Autodesk Inventor part; units mm, degrees
ref_plane "YZ Plane" through (0, 0, 0) normal (1, 0, 0) x (0, 1, 0)
ref_plane "XZ Plane" through (0, 0, 0) normal (0, 1, 0) x (-1, 0, 0)
ref_plane "XY Plane" through (0, 0, 0) normal (0, 0, 1) x (1, 0, 0)
sketch "Sketch1" plane through (0, 0, 0) normal (0, 0, 1) x (1, 0, 0)
  circle A0 centre (0, 0) radius 37.465
  dimension "d0" = 74.93
extrude "Extrusion1" add sketch "Sketch1" along normal blind 2.54
sketch "Sketch3" plane through (0, 0, 0) normal (0, 0, -1) x (-1, 0, 0)
  circle A0 centre (0, 0) radius 4.191
  circle A1 centre (0, 0) radius 7.9375
  circle A2 centre (0, 0) radius 2.3813
  dimension "d4" = 8.382
  dimension "d5" = 15.875
  dimension "d6" = 4.7625
extrude "Extrusion3" cut sketch "Sketch3" against normal through all contours A0 | A2
extrude "Extrusion4" add sketch "Sketch3" along normal blind 3.81 contours A1
sketch "Sketch4" plane through (0, 0, 2.54) normal (0, 0, 1) x (1, 0, 0)
  line L0 (0, 0) -> (0, 30.48)
  circle A0 centre (0, 30.48) radius 1.5875
  circle A1 centre (-26.3965, 15.24) radius 1.5875
  circle A2 centre (-26.3965, -15.24) radius 1.5875
  circle A3 centre (0, -30.48) radius 1.5875
  circle A4 centre (26.3965, -15.24) radius 1.5875
  circle A5 centre (26.3965, 15.24) radius 1.5875
  dimension "d13" = 30.48
  dimension "d14" = 3.175
  dimension "d17" = 360
extrude "Extrusion5" cut sketch "Sketch4" against normal blind 25.4
properties part number "SpoolEndFrontSide"
Part model, mm, in its own coordinate system. A direction names the side the tool comes from. Round coordinates to 2 decimals unless told otherwise and drop trailing zeros. Order: outer loops, then holes, each group sorted by start corner. A loop starts at its lowest first (then second) coordinate and runs counter-clockwise, first axis right, second up. Notation, with made-up numbers: M 26,21.25 L 40,21.25 A29 cw 40,51.25 Z; hole C -6.75,44 d9. An arc over 180 degrees is marked long. Put each result on its own line as item: value. Start each with the question number.
1. Drop flat-ended pins along their axis: pin 1 (12 mm diameter, centred on x = -8.5, y = -26.5, fed in from -Z); pin 2 (5 mm diameter, centred on x = 0, y = 30.48, fed in from +Z); pin 3 (3 mm diameter, centred on y = -3.5, z = 1, fed in from -X); pin 4 (3 mm diameter, centred on y = -15, z = 0, fed in from -X). Give the stop position or say it passes through.
2. Slice it at A-A on x = 0. List the corners of the cut face in (y, z) (1 decimal), then the cut area to 3 significant figures.
3. Slice it at C-C on y = -30.48. List the corners of the cut face in (x, z).
4. Slice it at D-D on y = 15.24. List the corners of the cut face in (x, z), then the cut area to 3 significant figures.
5. Tool access for faces 4 (the face through (26.1, -16.8, 1.3)), 5 (the face through (1.72, 7.75, -1.88)): list every direction of +Z, -Z, +X, -X, +Y, -Y with a clear straight run to the whole face (end or side of a thin tool).
6. Slice it at B-B on z = 1. List the corners of the cut face in (x, y) (1 decimal).
7. Drill centre lines: probe 1 along Y at (x, z) = (0, 0.5) (1 decimal); probe 2 along Z at (x, y) = (23, -11); probe 3 along Y at (x, z) = (1, 1.25). Where is each one in solid material? Low to high. Write a range as [from, to].
8. Two-plate mould, pull along Y, no slides. Class faces 1 (the face through (8, 1, 2.54)), 2 (the face through (-29.73, 22.8, 1.25)), 3 (the face through (-27.982, 15.31, 1.288)): +Y half, -Y half, draft (parallel to the pull), parting line (faces both ways), or undercut.
Findings:
1. pin 1: z = 0
1. pin 2: z = 2.54
1. pin 3: x = -37.41
1. pin 4: x = -34.95
2. outline: M -37.5,0 L -32.1,0 L -32.1,2.5 L -37.5,2.5 Z; M -28.9,0 L -7.9,0 L -7.9,-3.8 L -4.2,-3.8 L -4.2,2.5 L -28.9,2.5 Z; M 4.2,-3.8 L 7.9,-3.8 L 7.9,0 L 28.9,0 L 28.9,2.5 L 4.2,2.5 Z; M 32.1,0 L 37.5,0 L 37.5,2.5 L 32.1,2.5 Z
2. area: 181 mm2
3. outline: M -21.79,0 L -1.59,0 L -1.59,2.54 L -21.79,2.54 Z; M 1.59,0 L 21.79,0 L 21.79,2.54 L 1.59,2.54 Z
4. outline: M -34.23,0 L -27.98,0 L -27.98,2.54 L -34.23,2.54 Z; M -24.81,0 L 24.81,0 L 24.81,2.54 L -24.81,2.54 Z; M 27.98,0 L 34.23,0 L 34.23,2.54 L 27.98,2.54 Z
4. area: 158 mm2
5. face 4: +Z, -Z
5. face 5: -Z
6. outline: C 0,0 d74.9; hole C -26.4,-15.2 d3.2; hole C -26.4,15.2 d3.2; hole C 0,0 d8.4; hole C 0,-30.5 d3.2; hole C 0,30.5 d3.2; hole C 26.4,-15.2 d3.2; hole C 26.4,15.2 d3.2
7. probe 1: [-37.5, -32.1], [-28.9, -4.2], [4.2, 28.9], [32.1, 37.5]
7. probe 2: [0, 2.54]
7. probe 3: [-37.45, -31.71], [-29.25, -4.07], [4.07, 29.25], [31.71, 37.45]
8. face 1: draft
8. face 2: parting line
8. face 3: undercut
